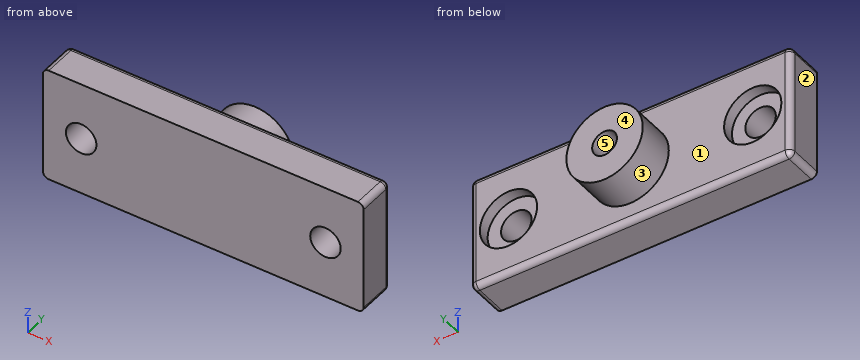
Autodesk Fusion 360 part; units mm, degrees
sketch "Sketch1" plane through (0, 0, 0) normal (0, 1, 0) x (1, 0, 0)
  line L0 (21, -7.5) -> (-21, -7.5)
  line L1 (-21, -7.5) -> (-21, 7.5)
  line L2 (-21, 7.5) -> (21, 7.5)
  line L3 (21, 7.5) -> (21, -7.5)
  dimension "d1" = 42
  dimension "d2" = 15
  dimension "d3" = 7.5
  dimension "d4" = 21
extrude "Extrude1" add sketch "Sketch1" along normal blind 5
sketch "Sketch2" plane through (0, 5, 0) normal (0, 1, 0) x (-1, 0, 0)
  line L0 (-21, -7.5) -> (21, -7.5)
  line L1 (21, -7.5) -> (21, 7.5)
  line L2 (21, 7.5) -> (-21, 7.5)
  line L3 (-21, 7.5) -> (-21, -7.5)
  circle A0 centre (0, 0) radius 5
  dimension "d7" = 10
extrude "Extrude2" add sketch "Sketch2" along normal blind 5 contours A0
sketch "Sketch3" plane through (0, 10, 0) normal (0, 1, 0) x (-1, 0, 0)
  circle A0 centre (0, 0) radius 5
  circle A1 centre (0, 0) radius 1.625
  dimension "d10" = 3.25
extrude "Extrude6" cut sketch "Sketch3" against normal blind 7.5 contours A1
sketch "Sketch7" plane through (0, 5, 0) normal (0, 1, 0) x (-1, 0, 0)
  circle A0 centre (0, 0) radius 5
  line L0 (-21, -7.5) -> (21, -7.5)
  line L1 (21, -7.5) -> (21, 7.5)
  line L2 (21, 7.5) -> (-21, 7.5)
  line L3 (-21, 7.5) -> (-21, -7.5)
  circle A1 centre (16, 0.0057) radius 2
  circle A2 centre (-16, 0.0028) radius 2
  dimension "d23" = 32
  dimension "d24" = 16
  dimension "d25" = 4
  dimension "d26" = 4
extrude "Extrude7" cut sketch "Sketch7" against normal through all contours A1 | A2
fillet "Fillet1" radius 0.75 8 edges at (0, 5, -7.5) (-21, 5, 0) (21, 5, 0) (0, 5, 7.5) (-21, 2.5, 7.5) (21, 2.5, 7.5) (21, 2.5, -7.5) (-21, 2.5, -7.5)
sketch "Sketch8" plane through (0, 5, 0) normal (0, 1, 0) x (-1, 0, 0)
  circle A0 centre (16, 0.0057) radius 2
  circle A1 centre (-16, 0.0028) radius 2
  circle A2 centre (16, 0.0057) radius 3.75
  circle A3 centre (-16, 0.0028) radius 3.75
  dimension "d29" = 7.5
  dimension "d30" = 7.5
extrude "Extrude8" cut sketch "Sketch8" against normal blind 1.5
Verification items for the finished model (mm, model axes). Face numbers are marked on the shaded views. A direction names the side the tool comes from. Coordinates: 2 decimals unless noted, no trailing zeros. Order: outer loops, then holes, each group sorted by start corner. A loop starts at its lowest first (then second) coordinate and runs counter-clockwise, first axis right, second up. Notation, with made-up numbers: (-3.75, 35) -> (29.25, 35) arc R13 cw to (29.25, 41) -> close; hole circle Ø6 at (3, 20.25). An arc over 180 degrees is marked (long way). Put each result on its own line as item: value. Start each with the question number.
1) Release check for a two-part mould opening along Z. For the marked faces 3, 4 and 5 record: pulls with the +Z half, pulls with the -Z half, needs draft (parallel to the pull), parting line crosses it, or undercut.
2) Cross-section at B-B (x = 0). Enter the section's corners in (y, z) (3 decimals), plus the area to 3 significant figures.
3) Material ranges on L1, parallel to Z at x = -16, y = 3.95; L2, parallel to Y at x = 10.5, z = 3.5; L3, parallel to X at y = 4.5, z = -3, recorded low to high.
4) Cross-section at A-A (x = -16). Enter the section's corners in (y, z).
5) Cross-section at C-C (y = 1.75). Enter the section's corners in (x, z).
6) Tool access check on the marked faces 1 and 2. Record the directions out of +Z, -Z, +X, -X, +Y, -Y that give a thin tool (end or side, any length) a straight path to the whole face; none if there is none.
7) Cross-section at D-D (z = -6.25). Enter the section's corners in (x, y), plus the area to 3 significant figures.
8) Go/stop test with flat-tipped pins: pin 1 (8.5 mm diameter, centred on x = 16, z = 0, fed in from +Y); pin 2 (1.9 mm diameter, centred on x = 0, z = 0, fed in from +Y); pin 3 (3.5 mm diameter, centred on x = -16, z = 0.01, fed in from -Y); pin 4 (2 mm diameter, centred on x = 9, y = 5.5, fed in from +Z). Record where each tip stops, or that it passes through.
Geometry check:
1. face 3: parting line crosses it
1. face 4: needs draft
1. face 5: undercut
2. outline: (0, -7.5) -> (4.25, -7.5) arc R0.75 ccw to (5, -6.75) -> (5, -5) -> (10, -5) -> (10, -1.625) -> (2.5, -1.625) -> (2.5, 1.625) -> (10, 1.625) -> (10, 5) -> (5, 5) -> (5, 6.75) arc R0.75 ccw to (4.25, 7.5) -> (0, 7.5) -> close
2. area: 100 mm^2
3. L1: z = -7.5 to -3.74, 3.76 to 7.5
3. L2: y = 0 to 5
3. L3: x = -20.96 to -18.24, -13.76 to 13.75, 18.25 to 20.96
4. outline: (0, -7.5) -> (4.25, -7.5) arc R0.75 ccw to (5, -6.75) -> (5, -3.74) -> (3.5, -3.74) -> (3.5, -1.99) -> (0, -1.99) -> close; (0, 2.01) -> (3.5, 2.01) -> (3.5, 3.76) -> (5, 3.76) -> (5, 6.75) arc R0.75 ccw to (4.25, 7.5) -> (0, 7.5) -> close
5. outline: (-21, -6.75) arc R0.75 ccw to (-20.25, -7.5) -> (20.25, -7.5) arc R0.75 ccw to (21, -6.75) -> (21, 6.75) arc R0.75 ccw to (20.25, 7.5) -> (-20.25, 7.5) arc R0.75 ccw to (-21, 6.75) -> close; hole circle Ø4 at (-16, 0.01); hole circle Ø4 at (16, 0)
6. face 1: +Y
6. face 2: +Z, -Z, -X, +Y, -Y
7. outline: (-21, 0) -> (21, 0) -> (21, 4.25) arc R0.75 ccw to (20.25, 5) -> (-20.25, 5) arc R0.75 ccw to (-21, 4.25) -> close
7. area: 210 mm^2
8. pin 1: stops at y = 5
8. pin 2: stops at y = 2.5
8. pin 3: passes through
8. pin 4: stops at z = 7.46
